The model under review builds one solid part; all positions refer to its coordinate system, in mm. Round coordinates to 2 decimals unless told otherwise and drop trailing zeros. Write each loop counter-clockwise with the first axis right and the second up, starting at its lowest first coordinate (ties: lowest second). Pieces come first, ordered by that corner, then holes.
Item 1: Add section D-D (x = 117.5). Give the boundary of the cut face in (y, z) (3 decimals).
Item 2: Draft analysis for pull direction X (two halves, no side actions). For faces 1 (the face through (241.231, 47.505, 1.565)), 2 (the face through (138, 113, 0)), state which applies: +X half, -X half, draft (parallel to the pull), parting line (faces both ways), or undercut.
Item 3: Clearance check with flat-ended pins moving along their axes: pin 1 Ø6.5 at (x, y) = (266.7, 266.7) entering from -Z; pin 2 Ø1 at (x, z) = (266.5, 2) entering from -Y. State where each tip first meets the part, or that it passes through.
Item 4: Add section A-A (x = 50.8). Give the boundary of the cut face in (y, z) (1 decimal).
Item 5: Add section C-C (z = 0.7). State how many separate pieces and enclosed holes the cut face has, plus the area to 3 significant figures.
Item 6: To check wall thickness, follow L1, parallel to Y at x = 266.7, z = 2.35; L2, parallel to X at y = -102.5, z = 1.8; L3, parallel to Y at x = 132.5, z = 1. State the ranges of each line that lie inside material, in increasing order.
Item 7: Add section B-B (y = 222). Give the boundary of the cut face in (x, z) (3 decimals), plus the area to 3 significant figures.
Autodesk Inventor part; units mm, degrees
ref_plane "YZ Plane" through (0, 0, 0) normal (1, 0, 0) x (0, 1, 0)
ref_plane "XZ Plane" through (0, 0, 0) normal (0, 1, 0) x (-1, 0, 0)
ref_plane "XY Plane" through (0, 0, 0) normal (0, 0, 1) x (1, 0, 0)
sketch "Sketch1" plane through (0, 0, 0) normal (0, 0, 1) x (1, 0, 0)
  line L0 (279.4, 279.4) -> (0, 279.4)
  line L1 (0, 279.4) -> (0, 0)
  circle A0 centre (50.8, 228.6) radius 14.2875
  circle A1 centre (50.8, 228.6) radius 250.0376 construction
  circle A2 centre (227.6033, 51.7967) radius 14.2875
  line L2 (50.8, 228.6) -> (279.4, 0) construction
  line L3 (279.4, 279.4) -> (279.4, -131.826)
  line L4 (279.4, -131.826) -> (253.746, -131.826)
  line L5 (253.746, -131.826) -> (253.746, -157.48)
  line L6 (253.746, -157.48) -> (241.3, -157.48)
  line L7 (241.3, -157.48) -> (241.3, -25.4)
  line L8 (241.3, -25.4) -> (87.1728, -25.4)
  line L9 (87.1728, -25.4) -> (87.1728, -157.48)
  line L10 (87.1728, -157.48) -> (0, -157.48)
  line L11 (0, -157.48) -> (0, 0)
  dimension "d5" = 500.0752
  dimension "d0" = 279.4
  dimension "d1" = 279.4
  dimension "d2" = 28.575
  dimension "d6" = 28.575
  dimension "d36" = 411.226
  dimension "d37" = 25.654
  dimension "d38" = 25.654
  dimension "d39" = 12.446
  dimension "d40" = 132.08
  dimension "d41" = 154.1272
extrude "Extrusion1" add sketch "Sketch1" along normal blind 3.175
sketch "Sketch2" plane through (0, 0, 3.175) normal (0, 0, 1) x (1, 0, 0)
  circle A0 centre (266.7, 12.7) radius 3.5687
  line L0 (0, 0) -> (279.4, 0)
  line L1 (279.4, 0) -> (279.4, 279.4)
  circle A1 centre (266.7, 76.2) radius 3.5687
  circle A2 centre (266.7, 139.7) radius 3.5687
  circle A3 centre (266.7, 203.2) radius 3.5687
  circle A4 centre (266.7, 266.7) radius 3.5687
  circle A5 centre (203.2, 12.7) radius 3.5687
  circle A6 centre (139.7, 12.7) radius 3.5687
  circle A7 centre (76.2, 12.7) radius 3.5687
  circle A8 centre (12.7, 12.7) radius 3.5687
  dimension "d9" = 7.1374
  dimension "d10" = 12.7
  dimension "d11" = 12.7
  dimension "d14" = 63.5
  dimension "d24" = 63.5
extrude "Extrusion2" cut sketch "Sketch2" against normal blind 3.175
sketch "Sketch3" plane through (0, 0, 3.175) normal (0, 0, 1) x (1, 0, 0)
  circle A0 centre (227.6033, 51.7967) radius 14.195
  circle A1 centre (209.6428, 69.7572) radius 2.0193
  circle A2 centre (245.5638, 33.8362) radius 2.0193
  line L0 (206.6033, 58.9967) -> (206.6033, 44.5967)
  line L1 (206.6033, 44.5967) -> (205.3783, 43.3717)
  line L2 (205.3783, 43.3717) -> (205.3783, 37.7967)
  line L3 (205.3783, 37.7967) -> (211.6033, 37.7967)
  arc A3 (213.6033, 35.7967) -> (211.6033, 37.7967) centre (211.6033, 35.7967) ccw
  line L4 (213.6033, 35.7967) -> (213.6033, 30.7967)
  line L5 (213.6033, 30.7967) -> (247.6033, 30.7967)
  arc A4 (247.6033, 30.7967) -> (248.6033, 31.7967) centre (227.6033, 51.7967) ccw
  line L6 (248.6033, 31.7967) -> (248.6033, 33.5967)
  line L7 (248.6033, 33.5967) -> (249.8283, 34.8217)
  line L8 (249.8283, 34.8217) -> (249.8283, 43.3717)
  line L9 (249.8283, 43.3717) -> (248.6033, 44.5967)
  line L10 (248.6033, 44.5967) -> (248.6033, 58.9967)
  line L11 (248.6033, 58.9967) -> (249.8283, 60.2217)
  line L12 (249.8283, 60.2217) -> (249.8283, 65.7967)
  line L13 (249.8283, 65.7967) -> (243.6033, 65.7967)
  arc A5 (241.6033, 67.7967) -> (243.6033, 65.7967) centre (243.6033, 67.7967) ccw
  line L14 (241.6033, 67.7967) -> (241.6033, 72.7967)
  line L15 (241.6033, 72.7967) -> (207.6033, 72.7967)
  arc A6 (207.6033, 72.7967) -> (206.6033, 71.7967) centre (227.6033, 51.7967) ccw
  line L16 (206.6033, 71.7967) -> (206.6033, 69.9967)
  line L17 (206.6033, 69.9967) -> (205.3783, 68.7717)
  line L18 (205.3783, 68.7717) -> (205.3783, 60.2217)
  line L19 (205.3783, 60.2217) -> (206.6033, 58.9967)
  circle A7 centre (227.6033, 51.7967) radius 14.2875
  point P0 (0, 0)
  dimension "d28" = 3.0395
  dimension "d29" = 4.2645
  dimension "d30" = 21
  dimension "d31" = 21
  dimension "d32" = 3.0395
  dimension "d33" = 4.2645
extrude "Extrusion3" cut sketch "Sketch3" against normal blind 25.4 contours A1 | A2
properties part number "1073-2017 Shooter Outside Plate Right"
Numbers:
1. outline: (-25.4, 0) - (279.4, 0) - (279.4, 3.175) - (-25.4, 3.175) - close
2. face 1: undercut
2. face 2: draft
3. pin 1: passes through
3. pin 2: stops at y = -131.83
4. outline: (-157.5, 0) - (214.3, 0) - (214.3, 3.2) - (-157.5, 3.2) - close; (242.9, 0) - (279.4, 0) - (279.4, 3.2) - (242.9, 3.2) - close
5. separate pieces: 1
5. enclosed holes: 13
5. area: 99,400 mm2
6. L1: y = -131.83 to 9.13, 16.27 to 72.63, 79.77 to 136.13, 143.27 to 199.63, 206.77 to 263.13, 270.27 to 279.4
6. L2: x = 0 to 87.17, 241.3 to 279.4
6. L3: y = -25.4 to 279.4
7. outline: (0, 0) - (38.128, 0) - (38.128, 3.175) - (0, 3.175) - close; (63.472, 0) - (279.4, 0) - (279.4, 3.175) - (63.472, 3.175) - close
7. area: 807 mm2
